Autodesk Inventor part; units mm, degrees
ref_plane "YZ Plane" through (0, 0, 0) normal (1, 0, 0) x (0, 1, 0)
ref_plane "XZ Plane" through (0, 0, 0) normal (0, 1, 0) x (-1, 0, 0)
ref_plane "XY Plane" through (0, 0, 0) normal (0, 0, 1) x (1, 0, 0)
sketch "Sketch1" plane through (0, 0, 0) normal (0, 0, 1) x (1, 0, 0)
  line L0 (0, 0) -> (1.5, 0)
  line L1 (1.5, 0) -> (1.5, 2)
  line L2 (1.5, 2) -> (0, 2)
  line L3 (0, 2) -> (0, 0)
  line L4 (0, 2) -> (3.5, 2)
  line L5 (3.5, 2) -> (3.5, 3)
  line L6 (3.5, 3) -> (0, 3)
  line L7 (0, 3) -> (0, 2)
  line L8 (0, 3) -> (2, 3)
  line L9 (2, 3) -> (2, 9.25)
  line L10 (2, 9.25) -> (0, 9.25)
  line L11 (0, 9.25) -> (0, 3)
  line L12 (0, 9.25) -> (1.5, 9.25)
  line L13 (1.5, 9.25) -> (1.5, 10.2)
  line L14 (1.5, 10.2) -> (0, 10.2)
  line L15 (0, 10.2) -> (0, 9.25)
  line L16 (0, 10.2) -> (2, 10.2)
  line L17 (2, 10.2) -> (2, 11)
  line L18 (2, 11) -> (0, 11)
  line L19 (0, 11) -> (0, 10.2)
  dimension "d8" = 4
  dimension "d9" = 3
  dimension "d10" = 8
  dimension "d11" = 9
  dimension "d12" = 11
  dimension "d13" = 0.8
  dimension "d14" = 1.75
  dimension "d16" = 7
revolve "Revolution1" add sketch "Sketch1" angle 360 about axis through (0, 9.25, 0) along (0, -1, 0)
properties part number "308-16" material "Steel"
The listing builds one solid part. Answer for the finished solid, in the listing's coordinates (mm). A direction names the side the tool comes from. Round coordinates to 2 decimals unless told otherwise and drop trailing zeros. Loops run counter-clockwise (first coordinate to the right, second up) from the corner with the lowest first, then second, coordinate; pieces in that order, holes last.
Q1. For a pull along Y with two mould halves and no side action, classify faces 1 (the face through (-1.5, 9.73, -0.07)), 2 (the face through (0, 0, 0)), 3 (the face through (-1.5, 1.01, -0.07)) as released by +Y, released by -Y, zero draft, split by the parting line, or undercut.
Q2. Which of the six approach directions +Z, -Z, +X, -X, +Y, -Y give full straight-line access (tool end or side, diameter ignored) to faces 4 (the face through (2, 3, -2)), 5 (the face through (3.233, 2.507, 1.341)), 6 (the face through (0, 2, -2))?
Q3. Section A-A, the plane x = 0 is taken. Determine the outline of the cut face in (y, z), then the cut area to 4 significant figures.
Q4. Given pin 1 Ø1 at (x, z) = (1, 3) entering from +Y; pin 2 Ø4 at (x, y) = (0.5, 9) entering from +Z; pin 3 Ø1 at (x, y) = (-1, 6) entering from +Z, each flat-ended and moving along its own axis, determine where each tip first touches the part or whether it passes through.
Q5. Find the intervals of material crossed by line 1 (Y direction, x = 0.5, z = 1.5); line 2 (Y direction, x = 2, z = 0.5); line 3 (X direction, y = 8.5, z = 1.5), in increasing order.
Q6. Section B-B, the plane z = 0 is taken. Determine the outline of the cut face in (x, y).
Q7. Section D-D, the plane x = 2.5 is taken. Determine the outline of the cut face in (y, z).
Q8. Section C-C, the plane y = 6.5 is taken. Determine the outline of the cut face in (x, z), then the cut area to 3 significant figures.
Completed:
1. face 1: undercut
1. face 2: released by -Y
1. face 3: zero draft
2. face 4: +Y
2. face 5: +Y, -Y
2. face 6: -Y
3. outline: (0, -1.5) - (2, -1.5) - (2, -3.5) - (3, -3.5) - (3, -2) - (9.25, -2) - (9.25, -1.5) - (10.2, -1.5) - (10.2, -2) - (11, -2) - (11, 2) - (10.2, 2) - (10.2, 1.5) - (9.25, 1.5) - (9.25, 2) - (3, 2) - (3, 3.5) - (2, 3.5) - (2, 1.5) - (0, 1.5) - close
3. area: 44.05 mm2
4. pin 1: stops at y = 3
4. pin 2: stops at z = 2
4. pin 3: stops at z = 1.94
5. line 1: y = 2 to 9.25, 10.2 to 11
5. line 2: y = 2 to 3
5. line 3: x = -1.32 to 1.32
6. outline: (-3.5, 2) - (-1.5, 2) - (-1.5, 0) - (1.5, 0) - (1.5, 2) - (3.5, 2) - (3.5, 3) - (2, 3) - (2, 9.25) - (1.5, 9.25) - (1.5, 10.2) - (2, 10.2) - (2, 11) - (-2, 11) - (-2, 10.2) - (-1.5, 10.2) - (-1.5, 9.25) - (-2, 9.25) - (-2, 3) - (-3.5, 3) - close
7. outline: (2, -2.45) - (3, -2.45) - (3, 2.45) - (2, 2.45) - close
8. outline: circle Ø4 at (0, 0)
8. area: 12.6 mm2
